Drawing for the job (mm, zero at the part's lowest x, y, z). A direction names the side the tool comes from. Coordinates: 2 decimals unless noted, no trailing zeros. Loops run counter-clockwise (first coordinate to the right, second up) from the corner with the lowest first, then second, coordinate; pieces in that order, holes last.
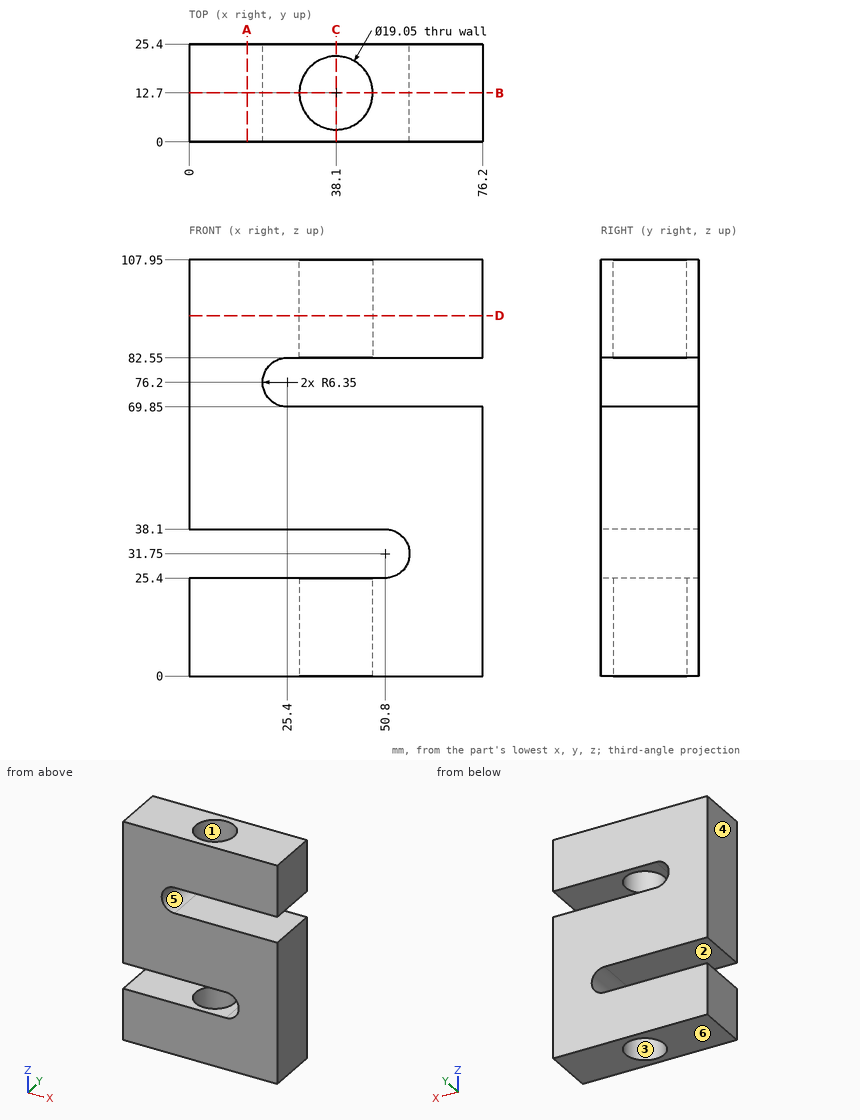
Q1. Saw through at C-C (x = 38.1). List the corners of the cut face in (y, z) (3 decimals), plus the area to 3 significant figures.
Q2. Drop flat-ended pins along their axis: P1, Ø8, axis at y = 9.5, z = 83, coming from the -X side; P2, Ø15, axis at x = 38.1, y = 12.7, coming from the -Z side. Give the stop position or say it passes through.
Q3. Mould opens along Z. For the marked faces 4, 5 and 6 say: released by +Z, released by -Z, zero draft, split by the parting line, or undercut.
Q4. Saw through at D-D (z = 93.5). List the corners of the cut face in (x, y) (3 decimals).
Q5. Tool access for the marked faces 1, 2 and 3: list every direction of +Z, -Z, +X, -X, +Y, -Y with a clear straight run to the whole face (end or side of a thin tool).
Q6. Probe line 1 (Z direction, x = 45, y = 1.75); line 2 (Y direction, x = 38.1, z = 101) (3 decimals); line 3 (Z direction, x = 9, y = 17.25). List the from-to ranges inside material, lowest first.
Q7. Saw through at A-A (x = 15). List the corners of the cut face in (y, z).
Q8. Saw through at B-B (y = 12.7). List the corners of the cut face in (x, z) (3 decimals).
Checked values:
1. outline: (0, 0) - (3.175, 0) - (3.175, 25.4) - (0, 25.4) - close; (0, 38.1) - (25.4, 38.1) - (25.4, 69.85) - (0, 69.85) - close; (0, 82.55) - (3.175, 82.55) - (3.175, 107.95) - (0, 107.95) - close; (22.225, 0) - (25.4, 0) - (25.4, 25.4) - (22.225, 25.4) - close; (22.225, 82.55) - (25.4, 82.55) - (25.4, 107.95) - (22.225, 107.95) - close
1. area: 1,130 mm2
2. P1: stops at x = 0
2. P2: stops at z = 38.1
3. face 4: zero draft
3. face 5: undercut
3. face 6: released by -Z
4. outline: (0, 0) - (76.2, 0) - (76.2, 25.4) - (0, 25.4) - close; hole circle Ø19.05 at (38.1, 12.7)
5. face 1: +Z
5. face 2: -X, +Y, -Y
5. face 3: -Z
6. line 1: z = 0 to 25.4, 38.1 to 69.85, 82.55 to 107.95
6. line 2: y = 0 to 3.175, 22.225 to 25.4
6. line 3: z = 0 to 25.4, 38.1 to 107.95
7. outline: (0, 0) - (25.4, 0) - (25.4, 25.4) - (0, 25.4) - close; (0, 38.1) - (25.4, 38.1) - (25.4, 107.95) - (0, 107.95) - close
8. outline: (0, 0) - (28.575, 0) - (28.575, 25.4) - (0, 25.4) - close; (0, 38.1) - (50.8, 38.1) arc R6.35 cw to (50.8, 25.4) - (47.625, 25.4) - (47.625, 0) - (76.2, 0) - (76.2, 69.85) - (25.4, 69.85) arc R6.35 cw to (25.4, 82.55) - (28.575, 82.55) - (28.575, 107.95) - (0, 107.95) - close; (47.625, 82.55) - (76.2, 82.55) - (76.2, 107.95) - (47.625, 107.95) - close
